The listing builds one solid part. Answer for the finished solid, in the listing's coordinates (mm). Face numbers are marked on the shaded views. A direction names the side the tool comes from. Give positions to 0.01 mm unless a question says otherwise; leave off trailing zeros. Write each loop counter-clockwise with the first axis right and the second up, starting at its lowest first coordinate (ties: lowest second). Pieces come first, ordered by that corner, then holes. Notation, with made-up numbers: M 81.5,-35.75 L 118.5,-35.75 A23 ccw 118.5,-27.75 Z; hole C -34,-6 d6. An arc over 180 degrees is marked long. Return JSON: item names as keys, results as strings.
from build123d import *

# Parameters (mm, degrees)
HOLE_WIZARD_M20_1_D           = 17.5
HOLE_WIZARD_M20_1_DEPTH       = 35
HOLE_WIZARD_M20_1_CSINK_D     = 20.05
HOLE_WIZARD_M20_1_CSINK_ANGLE = 90
HOLE_WIZARD_M20_1_TIP         = 5.257530416
CUT_EXTRUDE_START             = 19.5
CUT_EXTRUDE_1_DEPTH           = 171.181311678
SKETCH_5_R                    = 50.5
CUT_EXTRUDE_2_DEPTH           = 11.25
SKETCH_6_R                    = 36
CUT_EXTRUDE_3_DEPTH           = 19
SKETCH_7_R                    = 32.5
CUT_EXTRUDE_4_DEPTH           = 32.25
CHAMFER_1_SIZE                = 1
HOLE_WIZARD_1_D               = 38
HOLE_WIZARD_1_DEPTH           = 42.75
HOLE_WIZARD_1_TIP             = 11.416351762
HOLE_WIZARD_2_D               = 23


with BuildPart() as part:
    # 草图1 → 旋转1 (revolve)
    with BuildSketch(Plane(origin=(0, 0, 0), x_dir=(0, 0, -1), z_dir=(1, 0, 0)), mode=Mode.PRIVATE) as revolve_1_sk:
        Polygon((0, 0), (0, 83), (27, 83), (27, 53.624355653), (48, 41.5), (48, 30), (50.5, 30), (50.5, 25), (92.5, 25), (149, 22.038960471), (149, 0), align=None)
    revolve(revolve_1_sk.sketch.rotate(Axis((0, 0, 0), (0, 0, -1)), 90), axis=Axis((0, 0, 0), (0, 0, -1)))

    # M20 螺纹孔1
    with Locations(Plane(origin=(0, 0, -149), x_dir=(-1, 0, 0), z_dir=(0, 0, -1))):
        with Locations((0, 0)):
            CounterSinkHole(HOLE_WIZARD_M20_1_D / 2, HOLE_WIZARD_M20_1_CSINK_D / 2, depth=HOLE_WIZARD_M20_1_DEPTH, counter_sink_angle=HOLE_WIZARD_M20_1_CSINK_ANGLE)
            with Locations((0, 0, -(HOLE_WIZARD_M20_1_DEPTH + HOLE_WIZARD_M20_1_TIP / 2))):  # 118° drill point
                Cone(0, HOLE_WIZARD_M20_1_D / 2, HOLE_WIZARD_M20_1_TIP, mode=Mode.SUBTRACT)

    # 草图4 → 切除-拉伸1 (cut, through all)
    with BuildSketch(Plane(origin=(0, 0, 0), x_dir=(1, 0, 0), z_dir=(0, 1, 0)).offset(CUT_EXTRUDE_START)):
        with BuildLine():
            Line((7, 137), (7, 106))
            ThreePointArc((7, 106), (0, 99), (-7, 106))
            Line((-7, 106), (-7, 137))
            ThreePointArc((-7, 137), (0, 144), (7, 137))
        make_face()
    extrude(amount=CUT_EXTRUDE_1_DEPTH, mode=Mode.SUBTRACT)

    # 草图5 → 切除-拉伸2 (cut)
    with BuildSketch(Plane.XY):
        Circle(SKETCH_5_R)
    extrude(amount=-CUT_EXTRUDE_2_DEPTH, mode=Mode.SUBTRACT)

    # 草图6 → 切除-拉伸3 (cut)
    with BuildSketch(Plane.XY.offset(-11.25)):
        Circle(SKETCH_6_R)
    extrude(amount=-CUT_EXTRUDE_3_DEPTH, mode=Mode.SUBTRACT)

    # 草图7 → 切除-拉伸4 (cut)
    with BuildSketch(Plane.XY):
        Circle(SKETCH_7_R)
    extrude(amount=-CUT_EXTRUDE_4_DEPTH, mode=Mode.SUBTRACT)

    # 倒角1
    chamfer_1_edges = [part.edges().sort_by_distance(p)[0] for p in [
        (-50.5, 0, 0),
        (-36, 0, -11.25),
    ]]
    chamfer(chamfer_1_edges, length=CHAMFER_1_SIZE)

    # 孔1
    with Locations(Plane.XY):
        with Locations((0, 0)):
            Hole(HOLE_WIZARD_1_D / 2, depth=HOLE_WIZARD_1_DEPTH)
            with Locations((0, 0, -(HOLE_WIZARD_1_DEPTH + HOLE_WIZARD_1_TIP / 2))):  # 118° drill point
                Cone(0, HOLE_WIZARD_1_D / 2, HOLE_WIZARD_1_TIP, mode=Mode.SUBTRACT)

    # 孔2 (through all)
    with Locations(Plane(origin=(0, 0, -27), x_dir=(-1, 0, 0), z_dir=(0, 0, -1))):
        with Locations((-46.315494168, 46.315494168), (0, 65.5), (46.315494168, 46.315494168), (65.5, 0), (46.315494168, -46.315494168), (0, -65.5), (-46.315494168, -46.315494168), (-65.5, 0)):
            Hole(HOLE_WIZARD_2_D / 2)


solid = part.part
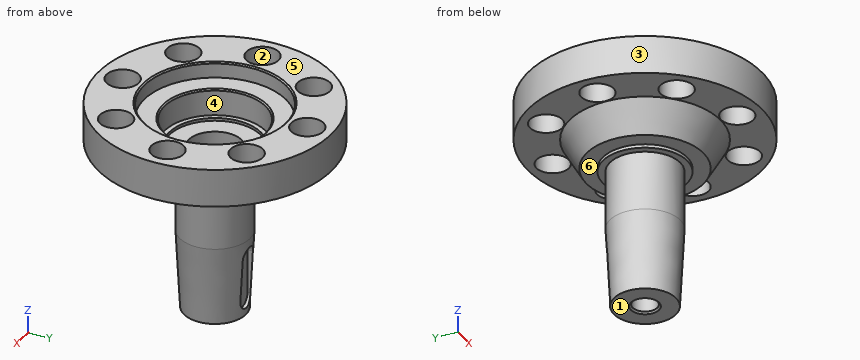
Item 1: A cutting plane is placed at D-D, the plane z = -38. Write down the section's boundary in (x, y).
Geometry results:
{"outline": "C 0,0 d94.55; hole C 0,0 d38"}
Item 2: Determine the mould class of the marked faces 1, 2 and 3 for opening direction X: +X half, -X half, draft (parallel to the pull), parting line (faces both ways), or undercut.
Geometry results:
{"face 1": "draft", "face 2": "undercut", "face 3": "parting line"}
Item 3: A cutting plane is placed at C-C, the plane z = -73.5. Write down the section's boundary in (x, y).
Geometry results:
{"outline": "C 0,0 d50"}
Item 4: Find the intervals of material crossed by line 1 (Y direction, x = 0, z = -9); line 2 (X direction, y = -44, z = -12.5); line 3 (Z direction, x = 69, y = -15.5), in increasing order.
Geometry results:
{"line 1": "y = -83 to -77, -54 to -50.5, 50.5 to 54, 77 to 83", "line 2": "x = -70.38 to -57.58, -35.05 to 35.05, 57.58 to 70.38", "line 3": "z = -27 to 0"}
Item 5: Given pin 1 Ø4 at (y, z) = (-6, -25.5) entering from -X; pin 2 Ø12 at (y, z) = (-22, -41.5) entering from +X; pin 3 Ø1.5 at (x, y) = (-48.5, -29) entering from -Z; pin 4 Ø18 at (x, y) = (-5.5, -6) entering from -Z, each flat-ended and moving along its own axis, determine where each tip first touches the part or whether it passes through.
Geometry results:
{"pin 1": "stops at x = -82.9", "pin 2": "stops at x = 44.37", "pin 3": "stops at z = -27", "pin 4": "stops at z = -149"}
Item 6: Which of the six approach directions +Z, -Z, +X, -X, +Y, -Y give full straight-line access (tool end or side, diameter ignored) to the marked faces 4, 5 and 6?
Geometry results:
{"face 4": "+Z", "face 5": "+Z, +X, -X, +Y, -Y", "face 6": "-Z"}
Item 7: A cutting plane is placed at A-A, the plane y = -65.5. Write down the section's boundary in (x, z), plus the area to 3 significant figures.
Geometry results:
{"outline": "M -50.98,-27 L -11.5,-27 L -11.5,0 L -50.98,0 Z; M 11.5,-27 L 50.98,-27 L 50.98,0 L 11.5,0 Z", "area": "2,130 mm2"}
